from build123d import *

# Parameters (mm, degrees)
SKETCH2_W           = 60
SKETCH2_H           = 42
SKETCH2_R           = 3.25
BOSS_EXTRUDE1_DEPTH = 8
SKETCH3_R           = 3.25
BOSS_EXTRUDE2_DEPTH = 8
FILLET1_R           = 3


with BuildPart() as part:
    # Sketch2 → Boss-Extrude1 (new body)
    with BuildSketch(Plane(origin=(0, 0, 0), x_dir=(1, 0, 0), z_dir=(0, 1, 0))):
        Rectangle(SKETCH2_W, SKETCH2_H)
        with Locations((-17.5, 0)):
            Circle(SKETCH2_R, mode=Mode.SUBTRACT)
        with Locations((17.5, 0)):
            Circle(SKETCH2_R, mode=Mode.SUBTRACT)
    extrude(amount=BOSS_EXTRUDE1_DEPTH)

    # Sketch3 → Boss-Extrude2 (add)
    with BuildSketch(Plane.XY.offset(21)):
        with BuildLine():
            Line((-7.5, 8), (-6.996052809, 23))
            ThreePointArc((-6.996052809, 23), (0, 29.764957256), (6.996052809, 23))
            Line((6.996052809, 23), (7.5, 8))
            Line((7.5, 8), (-7.5, 8))
        make_face()
        with Locations((0, 22.764957256)):
            Circle(SKETCH3_R, mode=Mode.SUBTRACT)
    boss_extrude2 = extrude(amount=-BOSS_EXTRUDE2_DEPTH)

    # Mirror1: Boss-Extrude2 across plane
    add(boss_extrude2.mirror(Plane.XY))

    # Fillet1
    fillet1_edges = [part.edges().sort_by_distance(p)[0] for p in [
        (-30, 8, 0),
        (0, 8, 13),
        (7.5, 8, 17),
        (-7.5, 8, 17),
        (0, 8, -13),
        (-7.5, 8, -17),
        (7.5, 8, -17),
        (30, 8, 0),
        (30, 4, 21),
        (-30, 4, 21),
        (-30, 4, -21),
        (30, 4, -21),
    ]]
    fillet(fillet1_edges, radius=FILLET1_R)


solid = part.part
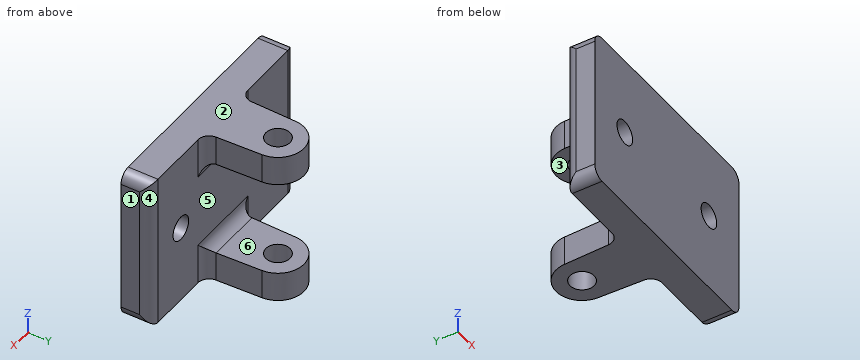
Geometry check sheet. Reference: the model listing, model coordinates, mm. Face numbers are marked on the shaded views. A direction names the side the tool comes from. Round coordinates to 2 decimals unless told otherwise and drop trailing zeros. Order: outer loops, then holes, each group sorted by start corner. A loop starts at its lowest first (then second) coordinate and runs counter-clockwise, first axis right, second up. Notation, with made-up numbers: M -27,88.5 L 8,88.5 A12 ccw 8,104.5 Z; hole C 73.25,78 d10. An arc over 180 degrees is marked long. Write each question's results on one line, items separated by ' | '. Start each with the question number.
1. Cross-section at B-B on y = 28. Record the boundary of the cut face in (x, z).
2. Material ranges on L1, parallel to Z at x = 5.5, y = 27; L2, parallel to X at y = 4, z = 0; L3, parallel to Y at x = 0, z = -16, recorded low to high. Write a range as from..to.
3. Cross-section at C-C on z = 0. Record the boundary of the cut face in (x, y).
4. Go/stop test with flat-tipped pins: P1, Ø8, axis at y = 14, z = 12, coming from the +X side; P2, Ø4, axis at x = -2.5, z = -8.5, coming from the +Y side. Record where each tip stops, or that it passes through.
5. Cross-section at A-A on x = 17.5. Record the boundary of the cut face in (y, z).
6. Draft check along Z on the marked faces 1, 2 and 3. Enter one of: pulls with the +Z half, pulls with the -Z half, needs draft (parallel to the pull), parting line crosses it, or undercut.
7. Cross-section at D-D on x = 0. Record the boundary of the cut face in (y, z), plus the area to 3 significant figures.
8. Set-up check for the marked faces 4, 5 and 6: record each of +Z, -Z, +X, -X, +Y, -Y from which the full face is reachable in a straight line by a thin tool's end or side.
Resolved:
1) outline: M -4.65,-21 L 4.65,-21 L 4.65,-13 L -4.65,-13 Z; M -4.65,13 L 4.65,13 L 4.65,21 L -4.65,21 Z
2) L1: -21..-13, 13..21 | L2: -30..-20.75, -14.25..14.25, 20.75..30 | L3: 0..19.51, 26.01..29.76
3) outline: M -30,0 L -20.75,0 L -20.75,8 L -27,8 A3 ccw -30,5 Z; M -14.25,0 L 14.25,0 L 14.25,8 L -14.25,8 Z; M 20.75,0 L 30,0 L 30,5 A3 ccw 27,8 L 20.75,8 Z
4) P1: x = 7.54 | P2: y = 8.04
5) outline: M 0,-21 L 8,-21 L 8,-3.25 L 0,-3.25 Z; M 0,3.25 L 8,3.25 L 8,21 L 0,21 Z
6) face 1: needs draft | face 2: pulls with the +Z half | face 3: undercut
7) outline: M 0,-21 L 19.51,-21 L 19.51,-13 L 11,-13 A3 cw 8,-10 L 8,10 A3 cw 11,13 L 19.51,13 L 19.51,21 L 0,21 Z; M 26.01,-21 L 29.76,-21 L 29.76,-13 L 26.01,-13 Z; M 26.01,13 L 29.76,13 L 29.76,21 L 26.01,21 Z | area: 584 mm2
8) face 4: +Z, -Z, +X, +Y | face 5: +Y | face 6: +X, -X, +Y
